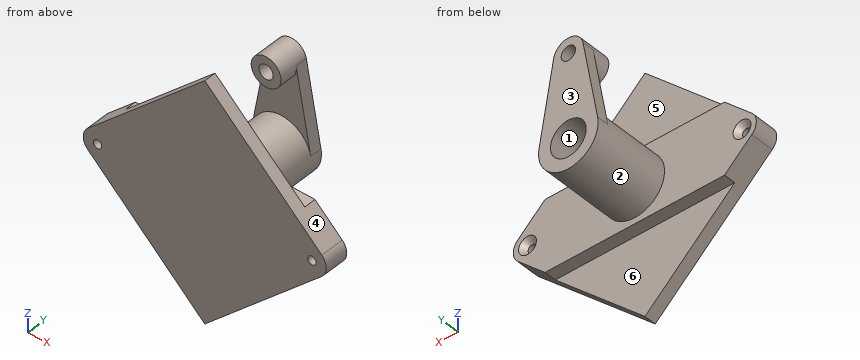
from build123d import *

# Parameters (mm, degrees)
SKETCH2_R                                           = 250
BOSS_EXTRUDE1_DEPTH                                 = 650
BOSS_EXTRUDE1_DEPTH_BACK                            = 200
SKETCH2_3_R                                         = 250
BOSS_EXTRUDE2_DEPTH                                 = 200
CUT_EXTRUDE1_DEPTH                                  = 100
BOSS_EXTRUDE4_DEPTH                                 = 100
SKETCH3_3_R                                         = 125
BOSS_EXTRUDE5_DEPTH                                 = 250
CSK_FOR_0_FLAT_HEAD_MACHINE_SCREW1_D                = 69.999999954
CSK_FOR_0_FLAT_HEAD_MACHINE_SCREW1_CSINK_D          = 149.999999974
CSK_FOR_0_FLAT_HEAD_MACHINE_SCREW1_CSINK_ANGLE      = 82
CBORE_FOR_0_BINDING_HEAD_MACHINE_SCREW1_D           = 80.00000002
CBORE_FOR_0_BINDING_HEAD_MACHINE_SCREW1_DEPTH       = 425.965575233
CBORE_FOR_0_BINDING_HEAD_MACHINE_SCREW1_CBORE_D     = 299.999999948
CBORE_FOR_0_BINDING_HEAD_MACHINE_SCREW1_CBORE_DEPTH = 350.000000024
CBORE_FOR_0_BINDING_HEAD_MACHINE_SCREW1_TIP         = 24.034424767
HOLE1_D                                             = 120
HOLE1_DEPTH                                         = 250


with BuildPart() as part:
    # Sketch2 → Boss-Extrude1 (new body, two sides)
    with BuildSketch(Plane(origin=(0, 0, 0), x_dir=(1, 0, 0), z_dir=(0, 1, 0))) as boss_extrude1_sk:
        Circle(SKETCH2_R)
    extrude(amount=BOSS_EXTRUDE1_DEPTH)
    extrude(boss_extrude1_sk.sketch, amount=-BOSS_EXTRUDE1_DEPTH_BACK)

    # Sketch2<3> → Boss-Extrude2 (add)
    with BuildSketch(Plane(origin=(0, 0, 0), x_dir=(1, 0, 0), z_dir=(0, 1, 0))):
        with BuildLine():
            Line((0, -1000), (981.679558011, -87.91160221))
            ThreePointArc((981.679558011, -87.91160221), (1020, 0), (981.679558011, 87.91160221))
            Line((981.679558011, 87.91160221), (0, 1000))
            Line((0, 1000), (-981.679558011, 87.91160221))
            ThreePointArc((-981.679558011, 87.91160221), (-1020, 0), (-981.679558011, -87.91160221))
            Line((-981.679558011, -87.91160221), (0, -1000))
        make_face()
        Circle(SKETCH2_3_R, mode=Mode.SUBTRACT)
    extrude(amount=-BOSS_EXTRUDE2_DEPTH)

    # Sketch2<5> → Cut-Extrude1 (cut)
    with BuildSketch(Plane(origin=(0, 0, 0), x_dir=(1, 0, 0), z_dir=(0, 1, 0))):
        Polygon((-753.409090909, -300), (0, -1000), (753.409090909, -300), align=None)
        Polygon((753.409090909, 300), (0, 1000), (-753.409090909, 300), align=None)
    extrude(amount=-CUT_EXTRUDE1_DEPTH, mode=Mode.SUBTRACT)

    # Sketch3 → Boss-Extrude4 (add)
    with BuildSketch(Plane(origin=(0, 650, 0), x_dir=(1, 0, 0), z_dir=(0, 1, 0))):
        with BuildLine():
            ThreePointArc((245.981737749, -44.642857143), (0, -250), (-245.981737749, -44.642857143))
            Line((-245.981737749, -44.642857143), (-122.990868875, -722.321428571))
            ThreePointArc((-122.990868875, -722.321428571), (-11.205833094, -575.503296009), (125, -700))
            ThreePointArc((125, -700), (124.496703991, -711.205833094), (122.990868875, -722.321428571))
            Line((122.990868875, -722.321428571), (245.981737749, -44.642857143))
        make_face()
    extrude(amount=-BOSS_EXTRUDE4_DEPTH)

    # Sketch3<3> → Boss-Extrude5 (add)
    with BuildSketch(Plane(origin=(0, 650, 0), x_dir=(1, 0, 0), z_dir=(0, 1, 0))):
        with Locations((0, -700)):
            Circle(SKETCH3_3_R)
    extrude(amount=-BOSS_EXTRUDE5_DEPTH)

    # CSK for #0 Flat Head Machine Screw1 (through all)
    with Locations(Plane(origin=(0, 0, 0), x_dir=(1, 0, 0), z_dir=(0, 1, 0))):
        with Locations((900, 0), (-900, 0)):
            CounterSinkHole(CSK_FOR_0_FLAT_HEAD_MACHINE_SCREW1_D / 2, CSK_FOR_0_FLAT_HEAD_MACHINE_SCREW1_CSINK_D / 2, counter_sink_angle=CSK_FOR_0_FLAT_HEAD_MACHINE_SCREW1_CSINK_ANGLE)

    # CBORE for #0 Binding Head Machine Screw1
    with Locations(Plane(origin=(0, 650, 0), x_dir=(1, 0, 0), z_dir=(0, 1, 0))):
        with Locations((0, 0)):
            CounterBoreHole(CBORE_FOR_0_BINDING_HEAD_MACHINE_SCREW1_D / 2, CBORE_FOR_0_BINDING_HEAD_MACHINE_SCREW1_CBORE_D / 2, CBORE_FOR_0_BINDING_HEAD_MACHINE_SCREW1_CBORE_DEPTH, depth=CBORE_FOR_0_BINDING_HEAD_MACHINE_SCREW1_DEPTH)
            with Locations((0, 0, -(CBORE_FOR_0_BINDING_HEAD_MACHINE_SCREW1_DEPTH + CBORE_FOR_0_BINDING_HEAD_MACHINE_SCREW1_TIP / 2))):  # 118° drill point
                Cone(0, CBORE_FOR_0_BINDING_HEAD_MACHINE_SCREW1_D / 2, CBORE_FOR_0_BINDING_HEAD_MACHINE_SCREW1_TIP, mode=Mode.SUBTRACT)

    # Hole1
    with Locations(Plane(origin=(0, 650, 0), x_dir=(1, 0, 0), z_dir=(0, 1, 0))):
        with Locations((0, -700)):
            Hole(HOLE1_D / 2, depth=HOLE1_DEPTH)


solid = part.part
Here's how the part is built. I have some questions about the finished solid (model axes, mm). Face numbers are marked on the shaded views. A direction names the side the tool comes from. Round coordinates to 2 decimals unless told otherwise and drop trailing zeros. Order: outer loops, then holes, each group sorted by start corner. A loop starts at its lowest first (then second) coordinate and runs counter-clockwise, first axis right, second up. Notation, with made-up numbers: (46.5, 3.5) -> (95.5, 3.5) arc R12 ccw to (95.5, 9.5) -> close; hole circle Ø2 at (-8.75, 36). An arc over 180 degrees is marked (long way). Return JSON: item names as keys, results as strings.
Q1. Which directions (+Z, -Z, +X, -X, +Y, -Y) give clear straight access to the entire face, cutting with the end or side of a thin tool? Please do the marked faces 1, 2 and 3.
Filled sheet:
{"face 1": "+Y", "face 2": "none", "face 3": "+Z, -Z, +X, -X, +Y"}
Q2. If we section it at D-D on x = 491: List the corners of the cut face in (y, z) for me.
Filled sheet:
{"outline": "(-200, -543.81) -> (-100, -543.81) -> (-100, -300) -> (0, -300) -> (0, 300) -> (-100, 300) -> (-100, 543.81) -> (-200, 543.81) -> close"}
Q3. If we section it at C-C on z = 671: List the corners of the cut face in (x, y) for me.
Filled sheet:
{"outline": "(-354.1, -200) -> (354.1, -200) -> (354.1, -100) -> (-354.1, -100) -> close; (-132.31, 550) -> (-121.59, 550) -> (-121.59, 400) -> (-52.53, 400) -> (-52.53, 650) -> (-132.31, 650) -> close; (52.53, 400) -> (121.59, 400) -> (121.59, 550) -> (132.31, 550) -> (132.31, 650) -> (52.53, 650) -> close"}
Q4. If we section it at B-B on x = -900: List the corners of the cut face in (y, z) for me, plus the area to 3 significant figures.
Filled sheet:
{"outline": "(-200, -163.8) -> (0, -163.8) -> (0, -75) -> (-46.01, -35) -> (-200, -35) -> close; (-200, 35) -> (-46.01, 35) -> (0, 75) -> (0, 163.8) -> (-200, 163.8) -> close", "area": "49,700 mm^2"}
Q5. For pin 1 Ø1.5 at (y, z) = (478.5, -146) entering from +X; pin 2 Ø8 at (x, y) = (63.5, 97.5) entering from +Z; pin 3 Ø1.5 at (x, z) = (-142, 790.5) entering from +Y, each with a flat end and sliding along its axis, tell me the tip position at first contact or that it passes through.
Filled sheet:
{"pin 1": "stops at x = 203.48", "pin 2": "stops at z = 242.82", "pin 3": "stops at y = -100"}
Q6. If we section it at A-A on y = 584: List the corners of the cut face in (x, z) for me, plus the area to 3 significant figures.
Filled sheet:
{"outline": "(-245.98, 44.64) arc R250 ccw (long way) to (245.98, 44.64) -> (122.99, 722.32) arc R125 ccw to (-122.99, 722.32) -> close; hole circle Ø300 at (0, 0); hole circle Ø120 at (0, 700)", "area": "307,000 mm^2"}
Q7. I need wall thicknesses on line 1 along Z through (x, y) = (0, 243); line 2 along X through (y, z) = (531, 700); line 3 along Z through (x, y) = (0, 380). Which ranges of each line are inside material? Lowest first, please. Write a range as from..to.
Filled sheet:
{"line 1": "z = -250..-40, 40..250", "line 2": "x = -125..-60, 60..125", "line 3": "z = -250..-150, 150..250"}
Q8. If we mould it in two halves opening along Y, with no side actions, what happens to the marked faces 4, 5 and 6? For each: released by +Y, released by -Y, zero draft, split by the parting line, or undercut.
Filled sheet:
{"face 4": "zero draft", "face 5": "undercut", "face 6": "released by +Y"}
